The listing builds one solid part. Answer for the finished solid, in the listing's coordinates (mm). A direction names the side the tool comes from. Coordinates: 2 decimals unless noted, no trailing zeros. Order: outer loops, then holes, each group sorted by start corner. A loop starts at its lowest first (then second) coordinate and runs counter-clockwise, first axis right, second up. Notation, with made-up numbers: (89, 64) - (94, 64) arc R12 ccw to (94, 78) - close; hole circle Ø2 at (53, 42). An arc over 180 degrees is marked (long way). One line per item, written item: value. Start each with the question number.
```python
from build123d import *
from OCP.BRepFilletAPI import BRepFilletAPI_MakeChamfer

# Parameters (mm, degrees)
SKETCH1_R           = 3.1
BOSS_EXTRUDE1_DEPTH = 9
SKETCH2_W           = 20
SKETCH2_H           = 40
CUT_EXTRUDE1_DEPTH  = 5
SKETCH3_R           = 6.05
CUT_EXTRUDE2_DEPTH  = 5
BOSS_EXTRUDE2_DEPTH = 35
SKETCH5_W           = 7
SKETCH5_H           = 12
CUT_EXTRUDE3_DEPTH  = 6
CHAMFER1_SIZE       = 6
CHAMFER1_SIZE2      = 4
CHAMFER2_SIZE       = 1
CUT_EXTRUDE4_DEPTH  = 12
CUT_EXTRUDE5_START  = -7
CUT_EXTRUDE5_DEPTH  = 11
SKETCH8_W           = 6
SKETCH8_H           = 6
BOSS_EXTRUDE3_DEPTH = 4
CHAMFER5_SIZE       = 4
CHAMFER5_SIZE_2     = 1
CHAMFER6_SIZE       = 1
CHAMFER6_SIZE2      = 4
CHAMFER7_SIZE       = 2.8
BOSS_EXTRUDE4_DEPTH = 6
CHAMFER8_START      = 16
CHAMFER8_DEPTH      = 0.515103423
CHAMFER8_START_2    = 16.515103423
CHAMFER8_2_DEPTH    = 6.413099807
CHAMFER8_START_3    = 11.656406461
CHAMFER8_3_DEPTH    = 6.343593539
CUT_EXTRUDE6_REACH  = 70.71
SKETCH10_R          = 1.55
CUT_EXTRUDE7_REACH  = 77.71
CUT_EXTRUDE7_START  = -7
SKETCH11_R          = 3.35
CHAMFER9_SIZE       = 1.8


with BuildPart() as part:
    # Sketch1 → Boss-Extrude1 (new body)
    with BuildSketch(Plane.XY):
        with BuildLine():
            Line((-10, 17), (-10, -17))
            ThreePointArc((-10, -17), (-9.121320344, -19.121320344), (-7, -20))
            Line((-7, -20), (10, -20))
            Line((10, -20), (25, -20))
            Line((25, -20), (38, -2))
            Line((38, -2), (45, -2))
            Line((45, -2), (45, -20))
            Line((45, -20), (57, -20))
            Line((57, -20), (57, 20))
            Line((57, 20), (-7, 20))
            ThreePointArc((-7, 20), (-9.121320344, 19.121320344), (-10, 17))
        make_face()
        with Locations((0, 10)):
            Circle(SKETCH1_R, mode=Mode.SUBTRACT)
        with Locations((0, -10)):
            Circle(SKETCH1_R, mode=Mode.SUBTRACT)
    extrude(amount=BOSS_EXTRUDE1_DEPTH)

    # Sketch2 → Cut-Extrude1 (cut)
    with BuildSketch(Plane.XY.offset(9)):
        Rectangle(SKETCH2_W, SKETCH2_H)
    extrude(amount=-CUT_EXTRUDE1_DEPTH, mode=Mode.SUBTRACT)

    # Sketch3 → Cut-Extrude2 (cut)
    with BuildSketch(Plane.XY.offset(9)):
        with Locations((28, -8)):
            Circle(SKETCH3_R)
    extrude(amount=-CUT_EXTRUDE2_DEPTH, mode=Mode.SUBTRACT)

    # Sketch4 → Boss-Extrude2 (add)
    with BuildSketch(Plane.XY.offset(9)):
        Polygon((45, -20), (57, -20), (57, 20), (10, 20), (10, 16.4), (45, 16.4), align=None)
    extrude(amount=BOSS_EXTRUDE2_DEPTH)

    # Sketch5 → Cut-Extrude3 (cut)
    with BuildSketch(Plane.XY.offset(9)):
        with Locations((41.5, 4)):
            Rectangle(SKETCH5_W, SKETCH5_H)
    extrude(amount=-CUT_EXTRUDE3_DEPTH, mode=Mode.SUBTRACT)

    # Chamfer1
    chamfer1_edges = [part.edges().sort_by_distance(p)[0] for p in [
        (41.5, 10, 9),
    ]]
    chamfer1_side = [part.faces().sort_by_distance(p)[0] for p in [
        (23.115817962, 1.462286031, 9),
    ]]
    chamfer(chamfer1_edges, length=CHAMFER1_SIZE, length2=CHAMFER1_SIZE2, reference=chamfer1_side[0])

    # Chamfer2
    chamfer2_edges = [part.edges().sort_by_distance(p)[0] for p in [
        (41.5, -2, 3),
    ]]
    chamfer(chamfer2_edges, length=CHAMFER2_SIZE)

    # Sketch6 → Cut-Extrude4 (cut)
    with BuildSketch(Plane(origin=(57, 0, 0), x_dir=(0, 0, -1), z_dir=(1, 0, 0))):
        with BuildLine():
            Line((-22, 11.05), (-44, 11.05))
            Line((-44, 11.05), (-44, -20))
            Line((-44, -20), (-14.055648488, -20))
            Line((-14.055648488, -20), (-14.055648488, -13.173106135))
            Line((-14.055648488, -13.173106135), (-11.317710156, -2.826868177))
            ThreePointArc((-11.317710156, -2.826868177), (-13.243876618, 6.740385992), (-22, 11.05))
        make_face()
        with BuildLine():
            Line((-40.5, 17.05), (-37.5, 17.05))
            ThreePointArc((-37.5, 17.05), (-35.95, 15.5), (-37.5, 13.95))
            Line((-37.5, 13.95), (-40.5, 13.95))
            ThreePointArc((-40.5, 13.95), (-42.05, 15.5), (-40.5, 17.05))
        make_face()
        with BuildLine():
            Line((-9.5, -17.05), (-6.5, -17.05))
            ThreePointArc((-6.5, -17.05), (-4.95, -15.5), (-6.5, -13.95))
            Line((-6.5, -13.95), (-9.5, -13.95))
            ThreePointArc((-9.5, -13.95), (-11.05, -15.5), (-9.5, -17.05))
        make_face()
    extrude(amount=-CUT_EXTRUDE4_DEPTH, mode=Mode.SUBTRACT)

    # Sketch7 → Cut-Extrude5 (cut)
    with BuildSketch(Plane(origin=(57, 0, 0), x_dir=(0, 0, -1), z_dir=(1, 0, 0)).offset(CUT_EXTRUDE5_START)):
        with BuildLine():
            Line((-6.5, -18.85), (-6.5, -20))
            Line((-6.5, -20), (-14.055648488, -20))
            Line((-14.055648488, -20), (-14.055648488, -12.15))
            Line((-14.055648488, -12.15), (-6.5, -12.15))
            ThreePointArc((-6.5, -12.15), (-3.15, -15.5), (-6.5, -18.85))
        make_face()
        with BuildLine():
            Line((-37.5, 18.85), (-40.5, 18.85))
            ThreePointArc((-40.5, 18.85), (-42.009108789, 18.490834443), (-43.194623608, 17.490352635))
            Line((-43.194623608, 17.490352635), (-44, 16.4))
            Line((-44, 16.4), (-44, 11.05))
            Line((-44, 11.05), (-37.5, 11.05))
            Line((-37.5, 11.05), (-37.5, 12.15))
            ThreePointArc((-37.5, 12.15), (-34.15, 15.5), (-37.5, 18.85))
        make_face()
    extrude(amount=-CUT_EXTRUDE5_DEPTH, mode=Mode.SUBTRACT)

    # Sketch8 → Boss-Extrude3 (add)
    with BuildSketch(Plane(origin=(0, 20, 0), x_dir=(1, 0, 0), z_dir=(0, 1, 0))):
        with Locations((54, -3)):
            Rectangle(SKETCH8_W, SKETCH8_H)
    extrude(amount=BOSS_EXTRUDE3_DEPTH)

    # Chamfer5
    chamfer5_edges_1 = [part.edges().sort_by_distance(p)[0] for p in [
        (51, 24, 3),
    ]]
    chamfer5_side_1 = [part.faces().sort_by_distance(p)[0] for p in [
        (51, 23.98, 3),
    ]]
    chamfer5_edges_2 = [part.edges().sort_by_distance(p)[0] for p in [
        (54, 24, 6),
    ]]
    chamfer5_side_2 = [part.faces().sort_by_distance(p)[0] for p in [
        (54, 24, 5.98),
    ]]
    chamfer5_edges_3 = [part.edges().sort_by_distance(p)[0] for p in [
        (57, 24, 3),
    ]]
    chamfer5_side_3 = [part.faces().sort_by_distance(p)[0] for p in [
        (56.98, 24, 3),
    ]]
    chamfer5 = BRepFilletAPI_MakeChamfer(part.part.solid().wrapped)
    for e in chamfer5_edges_1:
        chamfer5.Add(CHAMFER5_SIZE - 0.0001, CHAMFER5_SIZE_2 - 0.0001, e.wrapped, chamfer5_side_1[0].wrapped)
    for e in chamfer5_edges_2:
        chamfer5.Add(CHAMFER5_SIZE_2 - 0.0001, CHAMFER5_SIZE - 0.0001, e.wrapped, chamfer5_side_2[0].wrapped)
    for e in chamfer5_edges_3:
        chamfer5.Add(CHAMFER5_SIZE_2 - 0.0001, CHAMFER5_SIZE - 0.0001, e.wrapped, chamfer5_side_3[0].wrapped)
    add(Compound.cast(chamfer5.Shape()), mode=Mode.REPLACE)  # a hair under: the kernel refuses the full size

    # Chamfer6
    chamfer6_edges = [part.edges().sort_by_distance(p)[0] for p in [
        (38, 7, 9),
    ]]
    chamfer6_side = [part.faces().sort_by_distance(p)[0] for p in [
        (22.148058049, 0.854930368, 9),
    ]]
    chamfer(chamfer6_edges, length=CHAMFER6_SIZE, length2=CHAMFER6_SIZE2, reference=chamfer6_side[0])

    # Chamfer7
    chamfer7_edges = [part.edges().sort_by_distance(p)[0] for p in [
        (-3.1, 10, 0),
        (-3.1, -10, 0),
    ]]
    chamfer(chamfer7_edges, length=CHAMFER7_SIZE)

    # Sketch9 → Boss-Extrude4 (add)
    with BuildSketch(Plane.ZY.offset(-10)):
        with BuildLine():
            Line((44, 16.4), (44, 10))
            ThreePointArc((44, 10), (40.913417162, 5.380602337), (35.464466094, 6.464466094))
            Line((35.464466094, 6.464466094), (25.528932188, 16.4))
            Line((25.528932188, 16.4), (44, 16.4))
        make_face()
    extrude(amount=-BOSS_EXTRUDE4_DEPTH)

    # Chamfer8: read off the stored shape, not the designer's step
    # Chamfer8 outline → Chamfer8 (add)
    with BuildSketch(Plane.YZ.offset(CHAMFER8_START)):
        with BuildLine():
            ThreePointArc((10, 44), (5.380602337, 40.913417162), (6.464466094, 35.464466094))
            Line((6.464466094, 35.464466094), (16.4, 25.528932188))
            Line((16.4, 25.528932188), (16.4, 44))
            Line((16.4, 44), (10, 44))
        make_face()
    extrude(amount=CHAMFER8_DEPTH)

    # Chamfer8 2 outline → Chamfer8 2 (add)
    with BuildSketch(Plane.YZ.offset(CHAMFER8_START_2)):
        with BuildLine():
            ThreePointArc((10, 44), (5.380602337, 40.913417162), (6.464466094, 35.464466094))
            Line((6.464466094, 35.464466094), (16.4, 25.528932188))
            Line((16.4, 25.528932188), (16.4, 44))
            Line((16.4, 44), (10, 44))
        make_face()
    extrude(amount=CHAMFER8_2_DEPTH)

    # Chamfer8 3 outline → Chamfer8 3 (cut)
    with BuildSketch(Plane(origin=(0, 0, 0), x_dir=(0.500000000000006, 0.8660254037844353, 0), z_dir=(0.8660254037844352, -0.5000000000000061, 0)).offset(CHAMFER8_START_3)):
        with BuildLine():
            add(Edge.make_bspline(
                [(14.194351887, 35.464466094), (4.33836629, 44), (18.276834792, 44)],
                knots=[5.497787144, 5.497787144, 5.497787144, 7.853981634, 7.853981634, 7.853981634], degree=2, weights=[1, 0.382683432, 1]))
            Line((14.194351887, 35.464466094), (25.666918237, 25.528932188))
            Line((25.666918237, 25.528932188), (25.666918237, 44))
            Line((25.666918237, 44), (18.276834792, 44))
        make_face()
    extrude(amount=CHAMFER8_3_DEPTH, mode=Mode.SUBTRACT)

    # Cut-Extrude6: up to this plane
    cut_extrude6_end = Plane(origin=(22.92820323, 16.4, 44), z_dir=(-0.8660254037844355, 0.5000000000000057, 0))
    # Sketch10 → Cut-Extrude6 (cut, up to the surface)
    with BuildSketch(Plane.ZY.offset(-10), mode=Mode.PRIVATE) as cut_extrude6_sk1:
        with Locations(Location((39, 10, 0), (0, 0, 270))):
            Circle(SKETCH10_R)
    cut_extrude6_tool1 = split(extrude(cut_extrude6_sk1.sketch, amount=-CUT_EXTRUDE6_REACH, mode=Mode.PRIVATE), bisect_by=cut_extrude6_end, keep=Keep.BOTH, mode=Mode.PRIVATE)
    add(cut_extrude6_tool1.solids().sort_by_distance((10, 10, 39))[0], mode=Mode.SUBTRACT)

    # Sketch11 → Cut-Extrude7 (cut, up to next)
    with BuildSketch(Plane.ZY.offset(-10).offset(CUT_EXTRUDE7_START), mode=Mode.PRIVATE) as cut_extrude7_sk1:
        with Locations(Location((39, 10, 0), (0, 0, 270))):
            Circle(SKETCH11_R)
    cut_extrude7_tool1 = extrude(cut_extrude7_sk1.sketch, amount=-CUT_EXTRUDE7_REACH, mode=Mode.PRIVATE) & part.part
    add(cut_extrude7_tool1.solids().sort_by_distance((17, 10, 39))[0], mode=Mode.SUBTRACT)

    # Chamfer9
    chamfer9_edges = [part.edges().sort_by_distance(p)[0] for p in [
        (17, 11.55, 39),
    ]]
    chamfer(chamfer9_edges, length=CHAMFER9_SIZE - 0.0001)  # a hair under: the kernel refuses the full size


solid = part.part
```
(1) The part is cut by section C-C on y = -10. Determine the outline of the cut face in (x, z).
(2) The part is cut by section A-A on x = 43.5. Determine the outline of the cut face in (y, z).
(3) For faces 5 (the face through (20.78, 12.68, 35.49)), 6 (the face through (44.58, 18.5, 41.99)), 7 (the face through (54, -13.95, 8)), determine the directions among +Z, -Z, +X, -X, +Y, -Y from which every point of the face is accessible in a straight line to the end or side of a thin tool.
(4) The part is cut by section B-B on z = 39. Count the separate pieces of the cut face and the enclosed holes in it, plus the area to 3 significant figures.
(5) Flat-ended cylindrical pins translate along their axes: pin 1 Ø4 at (y, z) = (15.5, 39.5) entering from -X; pin 2 Ø1.6 at (x, z) = (41.5, 4.5) entering from -Y; pin 3 Ø16 at (x, y) = (0.5, 9.5) entering from +Z; pin 4 Ø8 at (x, z) = (2.5, 18) entering from +Y. Find the tip coordinate at first contact, or state that the pin passes through.
(6) The part is cut by section D-D on y = 3. Determine the outline of the cut face in (x, z).
(7) Consider probe 1 along Y at (x, z) = (0, 3.6); probe 2 along Z at (x, y) = (11, 10); probe 3 along Z at (x, y) = (20.5, -18). Determine where each line is inside the solid, lowest interval first.
(8) For a pull along X with two mould halves and no side action, classify faces 1 (the face through (57, 9, 13)), 2 (the face through (15.313, 10.216, 40.648)), 3 (the face through (54, 17.05, 39)), 4 (the face through (10, 18, 21)) as pulls with the +X half, pulls with the -X half, needs draft (parallel to the pull), parting line crosses it, or undercut.
Completed:
1. outline: (-10, 0) - (-5.9, 0) - (-3.1, 2.8) - (-3.1, 4) - (-10, 4) - close; (3.1, 2.8) - (5.9, 0) - (32.22, 0) - (32.22, 4) - (22.29, 4) - (22.29, 9) - (10, 9) - (10, 4) - (3.1, 4) - close; (45, 0) - (57, 0) - (57, 13.22) - (45, 13.22) - close
2. outline: (-2, 0) - (20, 0) - (20, 44) - (16.4, 44) - (17.49, 43.19) arc R3.35 cw to (18.85, 40.5) - (18.85, 37.5) arc R3.35 cw to (16.4, 34.27) - (16.4, 9) - (16, 9) - (10, 5) - (10, 3) - (-1, 3) - (-2, 2) - close
3. face 5: +Z, -Y
3. face 6: -Y
3. face 7: +X
4. separate pieces: 3
4. enclosed holes: 0
4. area: 228 mm2
5. pin 1: stops at x = 10
5. pin 2: stops at y = 10
5. pin 3: stops at z = 4
5. pin 4: passes through
6. outline: (-10, 0) - (57, 0) - (57, 11.37) - (45, 11.37) - (45, 3) - (38, 3) - (38, 5) - (37, 9) - (10, 9) - (10, 4) - (-10, 4) - close
7. probe 1: y = -20 to -13.1, -6.9 to 6.9, 13.1 to 20
7. probe 2: z = 0 to 9, 31.93 to 37.45, 40.55 to 44
7. probe 3: z = 0 to 9
8. face 1: pulls with the +X half
8. face 2: undercut
8. face 3: needs draft
8. face 4: pulls with the -X half
